Here's how the part is built. I have some questions about the finished solid (model axes, mm). A direction names the side the tool comes from. Round coordinates to 2 decimals unless told otherwise and drop trailing zeros. Write each loop counter-clockwise with the first axis right and the second up, starting at its lowest first coordinate (ties: lowest second). Pieces come first, ordered by that corner, then holes. Notation, with made-up numbers: (74, -22) - (88, -22) arc R19 cw to (88, 11) - close; hole circle Ø10 at (30.5, -22). An arc over 180 degrees is marked (long way). Write item = value, one per line. Start each with the question number.
Item 1: If we section it at B-B (y = 1): Please give me the cut outline in (x, z).
Item 2: If I drill on line 1 along Z through (x, y) = (3.5, -3); line 2 along Z through (x, y) = (3.75, -0.75); line 3 along Z through (x, y) = (12.75, 3.75), over which ranges is the centre line in solid material (lowest first)? Write a range as [from, to].
Item 3: Which directions (+Z, -Z, +X, -X, +Y, -Y) give clear straight access to the entire face, cutting with the end or side of a thin tool? Please do faces 1 (the face through (16.46, -0.94, 11.41)), 2 (the face through (2.5, 0, 0)), 3 (the face through (3, 0, 3)).
Item 4: If we section it at D-D (y = 3.5): Please give me the cut outline in (x, z).
Item 5: If we section it at C-C (y = -4): Please give me the cut outline in (x, z), and give its area (3 significant figures).
Item 6: Thinking about a two-plate mould opening in Z: for faces 4 (the face through (3, 0, -3)), 5 (the face through (10.709, -0.063, 4.245)), 6 (the face through (9, 4.5, 2)), which applies, pulls with the +Z half, pulls with the -Z half, needs draft (parallel to the pull), parting line crosses it, or undercut?
Item 7: For P1, Ø3, axis at y = -2.5, z = 5.5, coming from the -X side; P2, Ø1.5, axis at x = 11, z = 8, coming from the +Y side; P3, Ø5, axis at x = 17, z = 8, coming from the -Y side; P4, Ø4.5, axis at x = 4, y = -2, coming from the +Z side, each with a flat end and sliding along its axis, tell me the tip position at first contact or that it passes through.
Item 8: If we section it at A-A (x = 1): Please give me the cut outline in (y, z).
```python
from build123d import *
from build123d.topology import SkipClean

# Parameters (mm, degrees)
SKETCH_1_R      = 4.5
EXTRUDE_1_DEPTH = 3
EXTRUDE_2_DEPTH = 2.5
EXTRUDE_3_DEPTH = 2.5
LOFT_START      = -4.5
LOFT_1_DEPTH    = 9
SKETCH_4_R      = 2.9
EXTRUDE_5_DEPTH = 10
SKETCH_5_R      = 4.5
EXTRUDE_6_DEPTH = 1


# Read off the part's stored shape, not the designer's step: 放样1
with BuildPart() as part:
    # 草图1 → 凸台-拉伸1 (new, symmetric)
    with BuildSketch(Plane.XY):
        Circle(SKETCH_1_R)
        with BuildLine():
            Line((2.5, -1.833030278), (2.5, 1.833030278))
            ThreePointArc((2.5, 1.833030278), (-3.1, 0), (2.5, -1.833030278))
        make_face(mode=Mode.SUBTRACT)
    extrude(amount=EXTRUDE_1_DEPTH, both=True)

    # 草图2 → 凸台-拉伸2 (add, symmetric)
    with BuildSketch(Plane.XY):
        with BuildLine():
            ThreePointArc((4.5, 0), (3.181980515, -3.181980515), (0, -4.5))
            Line((0, -4.5), (10, -4.5))
            Line((10, -4.5), (10, 4.5))
            Line((10, 4.5), (0, 4.5))
            ThreePointArc((0, 4.5), (3.181980515, 3.181980515), (4.5, 0))
        make_face()
    extrude(amount=EXTRUDE_2_DEPTH, both=True)

    # 草图3 → 凸台-拉伸3 (add, symmetric)
    with BuildSketch(Plane(origin=(5, 0, -5), x_dir=(0, 1, 0), z_dir=(0.7071067811865438, 0, -0.7071067811865512))):
        with BuildLine():
            Line((-4.5, 7.071067812), (4.5, 7.071067812))
            Line((4.5, 7.071067812), (4.5, 16.771067812))
            ThreePointArc((4.5, 16.771067812), (0, 21.271067812), (-4.5, 16.771067812))
            Line((-4.5, 16.771067812), (-4.5, 7.071067812))
        make_face()
    extrude(amount=EXTRUDE_3_DEPTH, both=True)

    # 放样1 outline → 放样1 (add)
    with BuildSketch(Plane(origin=(0, 0, 0), x_dir=(1, 0, 0), z_dir=(0, 1, 0)).offset(LOFT_START)):
        Polygon((10, 0), (11.767766953, 1.767766953), (10, 2.5), align=None)
    extrude(amount=LOFT_1_DEPTH)

    # 草图4 → 凸台-拉伸5 (add)
    with BuildSketch(Plane(origin=(5, 0, -5), x_dir=(0, 1, 0), z_dir=(0.7071067811865438, 0, -0.7071067811865512))):
        with Locations(Location((0, 16.771067812, 0), (0, 0, 270))):
            Circle(SKETCH_4_R)
    extrude(amount=-EXTRUDE_5_DEPTH)

    # 草图5 → 凸台-拉伸6 (add)
    with SkipClean():  # the faces are left unmerged after this step: merging them gives an invalid solid
        with BuildSketch(Plane(origin=(3.232233047, 0, -3.232233047), x_dir=(0.7071067811865512, 0, 0.7071067811865438), z_dir=(-0.7071067811865438, 0, 0.7071067811865512))):
            with Locations((16.771067812, 0)):
                Circle(SKETCH_5_R)
        extrude(amount=EXTRUDE_6_DEPTH)
    add(part.part.scale(1), mode=Mode.REPLACE)  # the faces are merged on a copy


solid = part.part
```
Reply:
q1.outline = (-4.39, -3) - (-2.93, -3) - (-2.93, 3) - (-4.39, 3) - close; (2.5, -3) - (4.39, -3) - (4.39, -2.5) - (10, -2.5) - (11.77, -1.77) - (21.73, 8.19) - (17.49, 12.44) - (16.31, 11.26) - (11.71, 15.85) - (7.86, 12.01) - (12.46, 7.41) - (11.28, 6.23) - (11.99, 5.52) - (8.96, 2.5) - (4.39, 2.5) - (4.39, 3) - (2.5, 3) - close
q2.line_1 = [-2.5, 2.5]
q2.line_2 = [-3, 3]
q2.line_3 = [-0.79, 6.29], [7.45, 7.7]
q3.face_1 = none
q3.face_2 = +Z, -Z
q3.face_3 = +Z, -X, +Y, -Y
q4.outline = (-2.83, -3) - (2.83, -3) - (2.83, -2.5) - (10, -2.5) - (11.77, -1.77) - (20.63, 7.09) - (16.38, 11.33) - (12.38, 7.33) - (13.09, 6.63) - (8.96, 2.5) - (2.83, 2.5) - (2.83, 3) - (-2.83, 3) - close
q5.outline = (-2.06, -3) - (2.06, -3) - (2.06, -2.5) - (10, -2.5) - (11.77, -1.77) - (20.08, 6.55) - (15.84, 10.79) - (12.93, 7.88) - (13.63, 7.17) - (8.96, 2.5) - (2.06, 2.5) - (2.06, 3) - (-2.06, 3) - close
q5.area = 127 mm2
q6.face_4 = pulls with the -Z half
q6.face_5 = undercut
q6.face_6 = needs draft
q7.P1 = 10.46
q7.P2 = 1.31
q7.P3 = -4.5
q7.P4 = 3
q8.outline = (-4.5, -2.5) - (-4.39, -2.5) - (-4.39, -3) - (-2.93, -3) - (-2.93, 3) - (-4.39, 3) - (-4.39, 2.5) - (-4.5, 2.5) - close; (2.93, -3) - (4.39, -3) - (4.39, -2.5) - (4.5, -2.5) - (4.5, 2.5) - (4.39, 2.5) - (4.39, 3) - (2.93, 3) - close
